Autodesk Inventor part; units mm, degrees
ref_plane "YZ Plane" through (0, 0, 0) normal (1, 0, 0) x (0, 1, 0)
ref_plane "XZ Plane" through (0, 0, 0) normal (0, 1, 0) x (-1, 0, 0)
ref_plane "XY Plane" through (0, 0, 0) normal (0, 0, 1) x (1, 0, 0)
sketch "Sketch1" plane through (0, 0, 0) normal (0, 0, 1) x (1, 0, 0)
  line L0 (-4.1275, 8.1915) -> (4.1275, 8.1915)
  line L1 (-4.1275, 8.1915) -> (-4.1275, -8.1915)
  line L2 (-2.8575, -10.2235) -> (1.7145, -10.2235)
  line L3 (-2.8575, -10.2235) -> (-2.8575, -8.1915)
  line L4 (-2.8575, -8.1915) -> (-4.1275, -8.1915)
  line L5 (4.1275, 8.1915) -> (4.1275, 1.9685)
  line L6 (1.7145, -10.2235) -> (1.7145, 1.9685)
  line L7 (4.1275, 1.9685) -> (1.7145, 1.9685)
  point P0 (0, 0)
  point P1 (0, 8.1915)
  point P2 (-4.1275, 0)
  dimension "d0" = 8.255
  dimension "d2" = 1.27
  dimension "d3" = 2.032
  dimension "d4" = 18.415
  dimension "d5" = 4.572
  dimension "d6" = 6.223
extrude "Extrusion1" add sketch "Sketch1" along normal blind 31.6992
sketch "Sketch2" plane through (-4.1275, -8.1915, 31.6992) normal (-1, 0, 0) x (0, 0, 1)
  line L0 (-31.6992, 16.383) -> (0, 16.383)
  line L1 (-31.6992, 0) -> (-31.6992, 16.383)
  line L2 (-31.6992, 0) -> (0, 0)
  line L3 (-31.115, 16.383) -> (-28.2702, 16.383)
  line L4 (-28.2702, 14.097) -> (-28.2702, 0)
  line L5 (-28.2702, 0) -> (-31.115, 0)
  line L6 (-31.115, 0) -> (-31.115, 14.097)
  line L7 (-30.5054, 14.605) -> (-30.5054, 14.097)
  line L8 (-31.115, 16.383) -> (-30.5054, 14.605)
  line L9 (-30.5054, 14.097) -> (-31.115, 14.097)
  line L10 (-28.8798, 14.605) -> (-28.8798, 14.097)
  line L11 (-28.2702, 16.383) -> (-28.8798, 14.605)
  line L12 (-28.8798, 14.097) -> (-28.2702, 14.097)
  line L13 (-27.1526, 16.383) -> (-24.3078, 16.383)
  line L14 (-24.3078, 14.097) -> (-24.3078, 0)
  line L15 (-24.3078, 0) -> (-27.1526, 0)
  line L16 (-27.1526, 0) -> (-27.1526, 14.097)
  line L17 (-26.543, 14.605) -> (-26.543, 14.097)
  line L18 (-27.1526, 16.383) -> (-26.543, 14.605)
  line L19 (-26.543, 14.097) -> (-27.1526, 14.097)
  line L20 (-24.3078, 16.383) -> (-24.9174, 14.605)
  line L21 (-24.9174, 14.605) -> (-24.9174, 14.097)
  line L22 (-24.9174, 14.097) -> (-24.3078, 14.097)
  line L23 (-23.1902, 16.383) -> (-20.3454, 16.383)
  line L24 (-20.3454, 14.097) -> (-20.3454, 0)
  line L25 (-20.3454, 0) -> (-23.1902, 0)
  line L26 (-23.1902, 0) -> (-23.1902, 14.097)
  line L27 (-22.5806, 14.605) -> (-22.5806, 14.097)
  line L28 (-23.1902, 16.383) -> (-22.5806, 14.605)
  line L29 (-22.5806, 14.097) -> (-23.1902, 14.097)
  line L30 (-20.3454, 16.383) -> (-20.955, 14.605)
  line L31 (-20.955, 14.605) -> (-20.955, 14.097)
  line L32 (-20.955, 14.097) -> (-20.3454, 14.097)
  line L33 (-19.2278, 16.383) -> (-16.383, 16.383)
  line L34 (-16.383, 14.097) -> (-16.383, 0)
  line L35 (-16.383, 0) -> (-19.2278, 0)
  line L36 (-19.2278, 0) -> (-19.2278, 14.097)
  line L37 (-18.6182, 14.605) -> (-18.6182, 14.097)
  line L38 (-19.2278, 16.383) -> (-18.6182, 14.605)
  line L39 (-18.6182, 14.097) -> (-19.2278, 14.097)
  line L40 (-16.383, 16.383) -> (-16.9926, 14.605)
  line L41 (-16.9926, 14.605) -> (-16.9926, 14.097)
  line L42 (-16.9926, 14.097) -> (-16.383, 14.097)
  line L43 (-15.2654, 16.383) -> (-12.4206, 16.383)
  line L44 (-12.4206, 14.097) -> (-12.4206, 0)
  line L45 (-12.4206, 0) -> (-15.2654, 0)
  line L46 (-15.2654, 0) -> (-15.2654, 14.097)
  line L47 (-14.6558, 14.605) -> (-14.6558, 14.097)
  line L48 (-15.2654, 16.383) -> (-14.6558, 14.605)
  line L49 (-14.6558, 14.097) -> (-15.2654, 14.097)
  line L50 (-12.4206, 16.383) -> (-13.0302, 14.605)
  line L51 (-13.0302, 14.605) -> (-13.0302, 14.097)
  line L52 (-13.0302, 14.097) -> (-12.4206, 14.097)
  line L53 (-11.303, 16.383) -> (-8.4582, 16.383)
  line L54 (-8.4582, 14.097) -> (-8.4582, 0)
  line L55 (-8.4582, 0) -> (-11.303, 0)
  line L56 (-11.303, 0) -> (-11.303, 14.097)
  line L57 (-10.6934, 14.605) -> (-10.6934, 14.097)
  line L58 (-11.303, 16.383) -> (-10.6934, 14.605)
  line L59 (-10.6934, 14.097) -> (-11.303, 14.097)
  line L60 (-8.4582, 16.383) -> (-9.0678, 14.605)
  line L61 (-9.0678, 14.605) -> (-9.0678, 14.097)
  line L62 (-9.0678, 14.097) -> (-8.4582, 14.097)
  line L63 (-7.3406, 16.383) -> (-4.4958, 16.383)
  line L64 (-4.4958, 14.097) -> (-4.4958, 0)
  line L65 (-4.4958, 0) -> (-7.3406, 0)
  line L66 (-7.3406, 0) -> (-7.3406, 14.097)
  line L67 (-6.731, 14.605) -> (-6.731, 14.097)
  line L68 (-7.3406, 16.383) -> (-6.731, 14.605)
  line L69 (-6.731, 14.097) -> (-7.3406, 14.097)
  line L70 (-4.4958, 16.383) -> (-5.1054, 14.605)
  line L71 (-5.1054, 14.605) -> (-5.1054, 14.097)
  line L72 (-5.1054, 14.097) -> (-4.4958, 14.097)
  line L73 (-3.3782, 16.383) -> (-0.5334, 16.383)
  line L74 (-0.5334, 14.097) -> (-0.5334, 0)
  line L75 (-0.5334, 0) -> (-3.3782, 0)
  line L76 (-3.3782, 0) -> (-3.3782, 14.097)
  line L77 (-2.7686, 14.605) -> (-2.7686, 14.097)
  line L78 (-3.3782, 16.383) -> (-2.7686, 14.605)
  line L79 (-2.7686, 14.097) -> (-3.3782, 14.097)
  line L80 (-0.5334, 16.383) -> (-1.143, 14.605)
  line L81 (-1.143, 14.605) -> (-1.143, 14.097)
  line L82 (-1.143, 14.097) -> (-0.5334, 14.097)
  dimension "d9" = 0.5842
  dimension "d10" = 2.8448
  dimension "d11" = 0.6096
  dimension "d12" = 0.508
  dimension "d13" = 2.286
  dimension "d14" = 2.286
  dimension "d15" = 0.508
  dimension "d18" = 3.9624
extrude "Extrusion2" cut sketch "Sketch2" against normal blind 1.27 contours L0 L11 L10 L12 L4 L2 L6 L9 L7 L8 | L0 L20 L21 L22 L14 L2 L16 L19 L17 L18 | L0 L30 L31 L32 L24 L2 L26 L29 L27 L28 | L0 L40 L41 L42 L34 L2 L36 L39 L37 L38 | L0 L50 L51 L52 L44 L2 L46 L49 L47 L48 | L0 L60 L61 L62 L54 L2 L56 L59 L57 L58 | L0 L70 L71 L72 L64 L2 L66 L69 L67 L68 | L0 L80 L81 L82 L74 L2 L76 L79 L77 L78
properties part number "Connector, IDC, 8 Pin, SR"
Geometry: final body of the model. Coordinates: model frame, mm. A direction names the side the tool comes from. Round coordinates to 2 decimals unless told otherwise and drop trailing zeros. Loops run counter-clockwise (first coordinate to the right, second up) from the corner with the lowest first, then second, coordinate; pieces in that order, holes last. Notation, with made-up numbers: M 53.5,63.5 L 67.5,63.5 A16 cw 67.5,93.5 Z; hole C 59.25,58 d3. An arc over 180 degrees is marked long. Put each result on its own line as item: value. Start each with the question number.
(1) Material intervals for line 1 along X through (y, z) = (-2.75, 14); line 2 along X through (y, z) = (4.25, 10.5); line 3 along Y through (x, z) = (2.5, 12), sorted ascending. Write a range as [from, to].
(2) Section query C-C (x = 3). Return loops of the section in (y, z), then the cut area to 3 significant figures.
(3) Set-up query: faces 3 (the face through (-3.5, -8.192, 11.9)), 4 (the face through (-3.5, 7.31, 26.9)), 5 (the face through (-3.5, -1.2, 8.509)). Return all of +Z, -Z, +X, -X, +Y, -Y with unobstructed straight access to the full face (end or side cutting, diameter ignored); none if empty.
(4) Contact query for flat-ended pins moving along their axis: pin 1 Ø5 at (y, z) = (-6.5, 11.5) entering from +X; pin 2 Ø0.5 at (x, z) = (-3.5, 21) entering from -Y; pin 3 Ø0.6 at (x, z) = (-4, 8) entering from -Y; pin 4 Ø0.6 at (x, y) = (-3.5, 2) entering from -Z. Output: stop coordinate, or through.
(5) Section query A-A (z = 14). Return loops of the section in (x, y), then the cut area to 3 significant figures.
(6) Draft query along Z for faces 1 (the face through (-4.128, 0, 24)), 2 (the face through (-3.5, 7.31, 4.85)). Return one class per face: +Z half, -Z half, draft (parallel to the pull), parting line (faces both ways), or undercut.
(7) Section query B-B (x = -3.5). State how many separate pieces and enclosed holes the cut face has, then the cut area to 3 significant figures.
Findings below:
1. line 1: x = [-2.86, 1.71]
1. line 2: x = [-2.86, 4.13]
1. line 3: y = [1.97, 8.19]
2. outline: M 1.97,0 L 8.19,0 L 8.19,31.7 L 1.97,31.7 Z
2. area: 197 mm2
3. face 3: +Z, -Z, -X, -Y
3. face 4: -X, +Y
3. face 5: -X, -Y
4. pin 1: stops at x = 1.71
4. pin 2: stops at y = 5.91
4. pin 3: stops at y = -8.19
4. pin 4: stops at z = 0
5. outline: M -2.86,-10.22 L 1.71,-10.22 L 1.71,1.97 L 4.13,1.97 L 4.13,8.19 L -2.86,8.19 Z
5. area: 99.2 mm2
6. face 1: draft
6. face 2: undercut
7. separate pieces: 9
7. enclosed holes: 0
7. area: 160 mm2
